The listing builds one solid part. Answer for the finished solid, in the listing's coordinates (mm). Face numbers are marked on the shaded views. A direction names the side the tool comes from. Round coordinates to 2 decimals unless told otherwise and drop trailing zeros. Write each loop counter-clockwise with the first axis right and the second up, starting at its lowest first coordinate (ties: lowest second). Pieces come first, ordered by that corner, then holes. Notation, with made-up numbers: M 21,-4.75 L 25,-4.75 A19 cw 25,16.25 Z; hole C 5,11 d5. An arc over 180 degrees is marked long. Write each question's results on one line, items separated by ' | '.
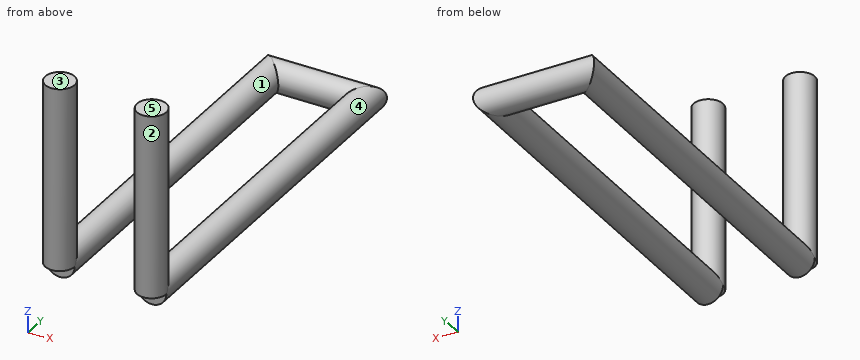
from build123d import *

# Parameters (mm, degrees)
F1_R     = 8
F3_DEPTH = 100
F2_R     = 8


with BuildPart() as f3:
    # F1 (on Top) → F3 (new body)
    with BuildSketch(Plane.XY):
        with Locations((-25, 0)):
            Circle(F1_R)
    extrude(amount=F3_DEPTH)



with BuildPart() as f3b:
    # F1 (on Top) → F3, piece 2 (new body)
    with BuildSketch(Plane.XY):
        with Locations((25, 0)):
            Circle(F1_R)
    extrude(amount=F3_DEPTH)


with BuildPart() as f3_1:
    add(f3.part)

    add(f3b.part)  # F4 merges F3b
    # F4: sweep along a path in F0
    with BuildLine(Plane.XY) as f4_path:
        Line((-25, 0), (-25, 200))
        Line((-25, 200), (0, 200))
        Line((0, 200), (25, 200))
        Line((25, 200), (25, 0))
    # F2 (on Front) → F4 (sweep)
    with BuildSketch(Plane.XZ):
        with Locations((-25, 0)):
            Circle(F2_R)
    sweep(path=f4_path.line, transition=Transition.RIGHT)


solid = f3_1.part
1) The mould has two halves that part along Y. Classify the marked faces 4 and 5: +Y half, -Y half, draft (parallel to the pull), parting line (faces both ways), or undercut.
Return value:
face 4: undercut | face 5: draft
2) Section B-B (z = 36.5) is taken. Determine the outline of the cut face in (x, y), then the cut area to 3 significant figures.
Return value:
outline: C -25,0 d16; C 25,0 d16 | area: 402 mm²
3) Section A-A (x = -25) is taken. Determine the outline of the cut face in (y, z), then the cut area to 3 significant figures.
Return value:
outline: M -8,0 L 0,0 L 0,-8 L 200,-8 A8 ccw 200,8 L 8,8 L 8,100 L -8,100 Z | area: 4,840 mm²
4) A tool of negligible diameter and unlimited length cuts with its end or side. For the marked faces 1, 2 and 3, from which of +Z, -Z, +X, -X, +Y, -Y can it reach the whole face along a straight path? Write none if from no direction.
Return value:
face 1: none | face 2: +Z | face 3: +Z, +X, -X, +Y, -Y
5) Find the intervals of material crossed by line 1 (Y direction, x = -24.5, z = 92); line 2 (Y direction, x = 19, z = 7); line 3 (X direction, y = 195.5, z = 2.5), in increasing order.
Return value:
line 1: -7.98 to 7.98 | line 2: -5.29 to 5.29, 196.13 to 203.87 | line 3: -32.6 to 32.6
6) Section D-D (y = 200) is taken. Determine the outline of the cut face in (x, z).
Return value:
outline: M -25,-8 L 25,-8 A8 ccw 25,8 L -25,8 A8 ccw Z
7) Each of these flat-tipped pins is pushed along its axis until it touches: pin 1 (10 mm diameter, centred on x = -9, z = 34.5, fed in from -Y); pin 2 (8 mm diameter, centred on x = -15, y = 111, fed in from +Z); pin 3 (10 mm diameter, centred on x = 14.5, z = 21.5, fed in from -Y); pin 4 (4 mm diameter, centred on x = -26.5, z = -3.5, fed in from -Y). Where does it stop, or does it pass through?
Return value:
pin 1: through | pin 2: z = 5.29 | pin 3: y = -5.81 | pin 4: y = 0
